The model under review builds one solid part; all positions refer to its coordinate system, in mm. Face numbers are marked on the shaded views. A direction names the side the tool comes from. Round coordinates to 2 decimals unless told otherwise and drop trailing zeros. Order: outer loops, then holes, each group sorted by start corner. A loop starts at its lowest first (then second) coordinate and runs counter-clockwise, first axis right, second up. Notation, with made-up numbers: M 65.5,4.5 L 94.5,4.5 A22 cw 94.5,39.5 Z; hole C 7,16 d4. An arc over 180 degrees is marked long. Use a Markdown table: item, result. Add a question column.
1. Consider section C-C on y = 4.75. State the section outline as (x, z) points.
2. To check wall thickness, follow probe 1 along Y at (x, z) = (3, 22.25); probe 2 along Z at (x, y) = (7.5, 3.5). State the ranges of each line that lie inside material, in increasing order.
3. For the marked faces 1 and 2, list the 3-axis set-ups (+Z, -Z, +X, -X, +Y, -Y) from which the entire face can be reached by the end or side of a thin tool; tool diameter is ignored.
4. Consider section D-D on z = 21.5. State the section outline as (x, y) points.
5. Consider section A-A on z = 13.25. State the section outline as (x, y) points.
6. Consider section B-B on x = 16. State the section outline as (y, z) points.
7. The part is to be moulded in two halves that separate along Y. For the marked faces 3, 4 and 5, say which applies: +Y half, -Y half, draft (parallel to the pull), parting line (faces both ways), or undercut.
8. Insertion check: P1, Ø14, axis at x = 16, y = 3, coming from the +Z side; P2, Ø2, axis at y = -9.5, z = 6, coming from the +X side. Each pin has a flat end and moves straight along its axis. Give the tip position at first contact, or say it passes through.
from build123d import *

# Parameters (mm, degrees)
F0_W     = 38.1
F0_H     = 25.4
F1_DEPTH = 12.7
F3_DEPTH = 12.7
F4_W     = 12.7
F4_H     = 12.7
F5_DEPTH = 50.8


with BuildPart() as f1:
    # F0 (on Front) → F1 (new body, symmetric)
    with BuildSketch(Plane.XZ):
        with Locations((19.05, 12.7)):
            Rectangle(F0_W, F0_H)
    extrude(amount=F1_DEPTH, both=True)

    # F2 (on Front) → F3 (cut, symmetric)
    with BuildSketch(Plane.XZ):
        Polygon((38.1, 25.4), (17.01173, 25.4), (38.1, 0), align=None)
    extrude(amount=F3_DEPTH, both=True, mode=Mode.SUBTRACT)

    # F4 (on Right) → F5 (cut)
    with BuildSketch(Plane.YZ):
        with Locations((0, 19.05)):
            Rectangle(F4_W, F4_H)
    extrude(amount=F5_DEPTH, mode=Mode.SUBTRACT)


solid = f1.part
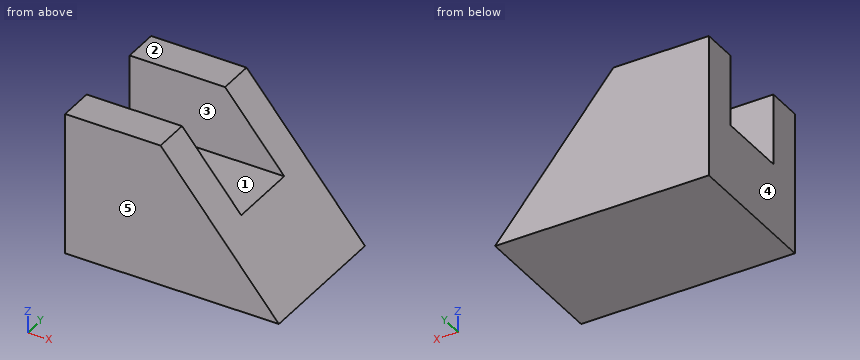
Answer block:
| question | item | result |
|---|---|---|
| 1 | outline | M 0,0 L 38.1,0 L 27.56,12.7 L 0,12.7 Z |
| 2 | probe 1 | -12.7 to -6.35, 6.35 to 12.7 |
| 2 | probe 2 | 0 to 12.7 |
| 3 | face 1 | +Z, +X, -X |
| 3 | face 2 | +Z, +X, -X, +Y, -Y |
| 4 | outline | M 0,-12.7 L 20.25,-12.7 L 20.25,-6.35 L 0,-6.35 Z; M 0,6.35 L 20.25,6.35 L 20.25,12.7 L 0,12.7 Z |
| 5 | outline | M 0,-12.7 L 27.1,-12.7 L 27.1,-6.35 L 0,-6.35 Z; M 0,6.35 L 27.1,6.35 L 27.1,12.7 L 0,12.7 Z |
| 6 | outline | M -12.7,0 L 12.7,0 L 12.7,25.4 L 6.35,25.4 L 6.35,12.7 L -6.35,12.7 L -6.35,25.4 L -12.7,25.4 Z |
| 7 | face 3 | undercut |
| 7 | face 4 | draft |
| 7 | face 5 | -Y half |
| 8 | P1 | z = 25.4 |
| 8 | P2 | x = 33.95 |
